Here's how the part is built. I have some questions about the finished solid (model axes, mm). Face numbers are marked on the shaded views. A direction names the side the tool comes from. Coordinates: 2 decimals unless noted, no trailing zeros. Loops run counter-clockwise (first coordinate to the right, second up) from the corner with the lowest first, then second, coordinate; pieces in that order, holes last. Notation, with made-up numbers: (3.25, 15) -> (20.25, 15) arc R22 ccw to (20.25, 28) -> close; hole circle Ø6 at (-18.75, 2.25). An arc over 180 degrees is marked (long way). Answer as a JSON object with one key per item and string values. Group by question number.
1) I'm going to push a flat-ended pin straight in: pin 1 (1.5 mm diameter, centred on y = 35, z = 40.5, fed in from +X). Where does the tip first touch, or does it pass through?
2) Which directions (+Z, -Z, +X, -X, +Y, -Y) give clear straight access to the entire face, cutting with the end or side of a thin tool? Please do the marked faces 1 and 2.
3) I want a section at C-C (y = 50). Write out the boundary of the cut face in (x, z), then the cut area to 3 significant figures.
4) I want a section at B-B (x = -645). Write out the boundary of the cut face in (y, z), then the cut area to 3 significant figures.
5) I want a section at A-A (z = 105). Write out the boundary of the cut face in (x, y), then the cut area to 3 significant figures.
6) If we mould it in two halves opening along X, with no side actions, what happens to the marked faces 3, 4 and 5? For each: +X half, -X half, draft (parallel to the pull), parting line (faces both ways), or undercut.
7) I need wall thicknesses on probe 1 along Y at (x, z) = (-841.5, 170.5); probe 2 along X at (y, z) = (66, 113); probe 3 along X at (y, z) = (72, 117.5). Which ranges of each line are inside material? Lowest first, please. Write a range as [from, to].
```python
from build123d import *

# Parameters (mm, degrees)
SKETCH2_R           = 50
SKETCH2_W           = 1100
SKETCH2_H           = 100
BOSS_EXTRUDE1_DEPTH = 250
SKETCH3_R           = 40
SKETCH3_W           = 1100
SKETCH3_H           = 80
CUT_EXTRUDE1_DEPTH  = 1182.101181102


with BuildPart() as part:
    # Sketch2 → Boss-Extrude1 (new body)
    with BuildSketch(Plane.XY):
        with Locations((-1100, 50)):
            Circle(SKETCH2_R)
        with Locations((0, 50)):
            Circle(SKETCH2_R)
        with Locations((-550, 50)):
            Rectangle(SKETCH2_W, SKETCH2_H)
    extrude(amount=BOSS_EXTRUDE1_DEPTH)

    # Sketch3 → Cut-Extrude1 (cut, through all)
    with BuildSketch(Plane.XY.offset(250)):
        with Locations((-1100, 50)):
            Circle(SKETCH3_R)
        with Locations((0, 50)):
            Circle(SKETCH3_R)
        with Locations((-550, 50)):
            Rectangle(SKETCH3_W, SKETCH3_H)
    extrude(amount=-CUT_EXTRUDE1_DEPTH, mode=Mode.SUBTRACT)


solid = part.part
```
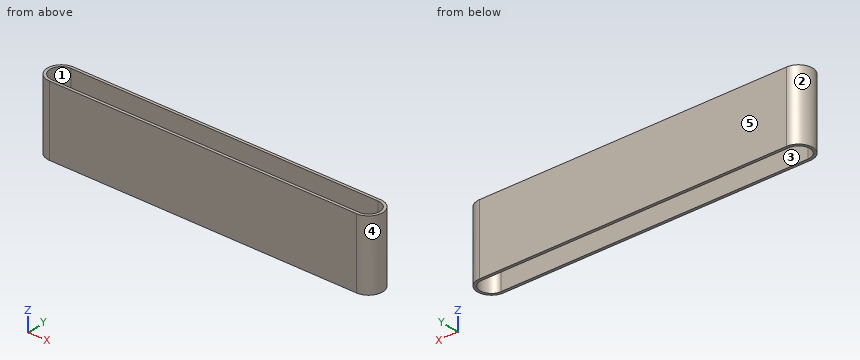
Determined:
{
 "1": {"pin 1": "x = 47.93"},
 "2": {"face 1": "+Z, -Z", "face 2": "+Z, -Z, -X"},
 "3": {"outline": "(-1150, 0) -> (-1140, 0) -> (-1140, 250) -> (-1150, 250) -> close; (40, 0) -> (50, 0) -> (50, 250) -> (40, 250) -> close", "area": "5,000 mm^2"},
 "4": {"outline": "(0, 0) -> (10, 0) -> (10, 250) -> (0, 250) -> close; (90, 0) -> (100, 0) -> (100, 250) -> (90, 250) -> close", "area": "5,000 mm^2"},
 "5": {"outline": "(-1100, 0) -> (0, 0) arc R50 ccw to (0, 100) -> (-1100, 100) arc R50 ccw to start; hole (-1100, 10) -> (0, 10) arc R40 ccw to (0, 90) -> (-1100, 90) arc R40 ccw to start", "area": "24,800 mm^2"},
 "6": {"face 3": "undercut", "face 4": "+X half", "face 5": "draft"},
 "7": {"probe 1": "[0, 10], [90, 100]", "probe 2": "[-1147.37, -1136.66], [36.66, 47.37]", "probe 3": "[-1144.9, -1133.41], [33.41, 44.9]"}
}
